Model file for the job. Use its own axes, mm. Face numbers are marked on the shaded views. A direction names the side the tool comes from. Give positions to 0.01 mm unless a question says otherwise; leave off trailing zeros. Loops run counter-clockwise (first coordinate to the right, second up) from the corner with the lowest first, then second, coordinate; pieces in that order, holes last. Notation, with made-up numbers: (-6.75, 19.5) -> (38.25, 19.5) arc R19 cw to (38.25, 23.5) -> close; hole circle Ø8 at (36.5, -28). An arc over 180 degrees is marked (long way). Use CSV: the item, a comma, the result in double quotes. Start each with the question number.
(1) Flat gauge pins, fed straight in: pin 1 (6 mm diameter, centred on y = -17, z = 13.5, fed in from -X); pin 2 (1.5 mm diameter, centred on x = 12.5, y = -13, fed in from +Z); pin 3 (10 mm diameter, centred on y = -8, z = 24.5, fed in from +X); pin 4 (9.5 mm diameter, centred on x = 0, z = 29, fed in from -Y). Where does each tip first touch, or does it go through?
(2) Pull direction Z, two halves, no side cores. Call the marked faces 5, 6, 7 and 8: pulls with the +Z half, pulls with the -Z half, needs draft (parallel to the pull), parting line crosses it, or undercut.
(3) 3-axis set-ups, long thin cutter, end or side, ignore diameter. For the marked faces 1, 2, 3 and 4: which of +Z, -Z, +X, -X, +Y, -Y reach the whole face in a straight line?
(4) Cut at B-B on y = 3. Write the cut outline in (x, z), then the cut area to 3 significant figures.
(5) Cut at A-A on x = 0. Write the cut outline in (y, z), then the cut area to 3 significant figures.
(6) Cut at D-D on z = 44.5. Write the cut outline in (x, y).
(7) Drill centre lines: probe 1 along X at (y, z) = (6.5, 35.5); probe 2 along Z at (x, y) = (0, -4.25); probe 3 along Y at (x, z) = (-29.5, 43). Where is each one in solid material? Low to high.
(8) Cut at C-C on z = 34. Write the cut outline in (x, y).
from build123d import *

# Parameters (mm, degrees)
F1_DEPTH    = 48
F2_DEPTH    = 10
F3_T1_DEPTH = 30
F4_T1_DEPTH = 30
F6_DEPTH    = 3
F5_W        = 28
F5_H        = 5
F7_DEPTH    = 5
F8_R        = 6
F9_R        = 6
F11_D       = 12


# Not quite as in the source:
# - a fillet or chamfer that OpenCascade refuses, or shapes differently, is made with other operations: its cross-section is extruded or revolved along the edge and cut away or added


with BuildPart() as f1:
    # F0 (on Top) → F1 (new body)
    with BuildSketch(Plane.XY):
        Polygon((-21, 20), (-31, 20), (-31, -10), (31, -10), (31, 20), (21, 20), (21, 0), (-21, 0), align=None)
    extrude(amount=F1_DEPTH)

    # F0 (on Top) → F2 (join)
    with BuildSketch(Plane.XY):
        Polygon((-31, 20), (-46, 20), (-46, -28), (46, -28), (46, 20), (31, 20), (31, -10), (-31, -10), align=None)
        Polygon((-21, 20), (-31, 20), (-31, -10), (31, -10), (31, 20), (21, 20), (21, 0), (-21, 0), align=None)
    extrude(amount=F2_DEPTH)

    # F3: fillet of radius 20 on 1 edges, made by hand

    # F3_s2 → F3_t1 (join)
    with BuildSketch(Plane.XZ.offset(-20)):
        with BuildLine():
            ThreePointArc((31, 29.364916731), (35.1886116992, 17.1174680171), (46, 10))
            Line((46, 10), (31, 10))
            Line((31, 10), (31, 29.364916731))
        make_face()
    extrude(amount=F3_T1_DEPTH)

    # F4: fillet of radius 20 on 1 edges, made by hand

    # F4_s2 → F4_t1 (join)
    with BuildSketch(Plane.XZ.offset(-20)):
        with BuildLine():
            ThreePointArc((-46, 10), (-35.1886116992, 17.1174680171), (-31, 29.364916731))
            Line((-31, 29.364916731), (-31, 10))
            Line((-31, 10), (-46, 10))
        make_face()
    extrude(amount=F4_T1_DEPTH)

    # F5 (on face) → F6 (join)
    with BuildSketch(Plane.XZ.offset(10)):
        with BuildLine():
            Line((-14, 29), (-14, 15))
            Line((-14, 15), (14, 15))
            Line((14, 15), (14, 29))
            ThreePointArc((14, 29), (0, 43), (-14, 29))
        make_face()
    extrude(amount=F6_DEPTH)

    # F5 (on face) → F7 (join)
    with BuildSketch(Plane.XZ.offset(10)):
        with Locations((0, 12.5)):
            Rectangle(F5_W, F5_H)
    extrude(amount=F7_DEPTH)

    # F8
    f8_edges = [f1.edges().sort_by_distance(p)[0] for p in [
        (46, -28, 5),
    ]]
    fillet(f8_edges, radius=F8_R)

    # F9
    f9_edges = [f1.edges().sort_by_distance(p)[0] for p in [
        (-46, -28, 5),
    ]]
    fillet(f9_edges, radius=F9_R)

    # F11 (through all)
    with Locations(Plane.XZ.offset(13)):
        with Locations((0, 29)):
            Hole(F11_D / 2)


solid = f1.part
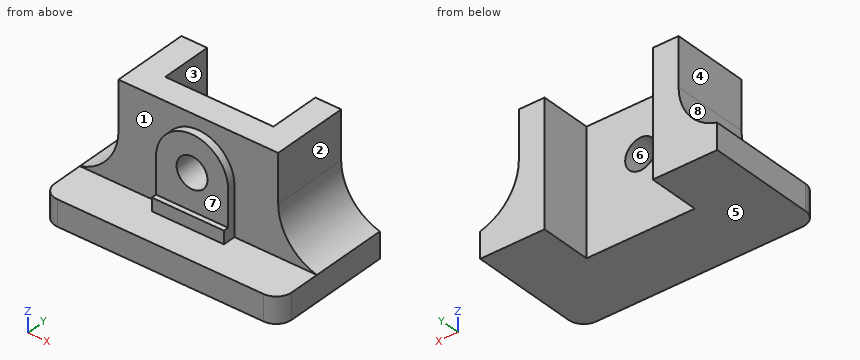
Check result:
1,pin 1,"x = -14"
1,pin 2,"z = 36.61"
1,pin 3,"x = 33.6"
1,pin 4,"through"
2,face 5,"pulls with the -Z half"
2,face 6,"undercut"
2,face 7,"needs draft"
2,face 8,"pulls with the +Z half"
3,face 1,"+Z, -Y"
3,face 2,"+Z, +X, +Y, -Y"
3,face 3,"+Z, -Z, +Y"
3,face 4,"+Z, -X, +Y, -Y"
4,outline,"(-46, 0) -> (-21, 0) -> (-21, 48) -> (-31, 48) -> (-31, 29.36) arc R20 cw to (-46, 10) -> close; (21, 0) -> (46, 0) -> (46, 10) arc R20 cw to (31, 29.36) -> (31, 48) -> (21, 48) -> close"
4,area,"1,410 mm²"
5,outline,"(-28, 0) -> (0, 0) -> (0, 23) -> (-13, 23) -> (-13, 15) -> (-15, 15) -> (-15, 10) -> (-28, 10) -> close; (-13, 35) -> (0, 35) -> (0, 48) -> (-10, 48) -> (-10, 43) -> (-13, 43) -> close"
5,area,"613 mm²"
6,outline,"(-31, -10) -> (31, -10) -> (31, 20) -> (21, 20) -> (21, 0) -> (-21, 0) -> (-21, 20) -> (-31, 20) -> close"
7,probe 1,"-31 to -21, 21 to 31"
7,probe 2,"0 to 23, 35 to 48"
7,probe 3,"-10 to 20"
8,outline,"(-31, -10) -> (-13.08, -10) -> (-13.08, -13) -> (-3.32, -13) -> (-3.32, 0) -> (-21, 0) -> (-21, 20) -> (-31, 20) -> close; (3.32, -13) -> (13.08, -13) -> (13.08, -10) -> (31, -10) -> (31, 20) -> (21, 20) -> (21, 0) -> (3.32, 0) -> close"
